Input: dimensioned drawing with shaded views. Units: mm. Origin: part minimum x, y, z. Round coordinates to 2 decimals unless told otherwise and drop trailing zeros. Loops run counter-clockwise (first coordinate to the right, second up) from the corner with the lowest first, then second, coordinate; pieces in that order, holes last. Notation, with made-up numbers: (42, 61.5) - (97, 61.5) arc R17 ccw to (97, 70.5) - close; hole circle Ø10 at (31.25, -0.75). An arc over 180 degrees is marked (long way). Answer as a JSON object with one key per item and string values. Group by question number.
Item 1: Line query: line 1 (Y direction, x = 29.5, z = 21.25) (1 decimal); line 2 (Y direction, x = 15.5, z = 11.75); line 3 (Y direction, x = 2.5, z = 3.5). Output: solid intervals per line, ascending.
Item 2: First-contact query: pin 1 (1.5 mm diameter, centred on x = 25.5, z = 8, fed in from +Y); pin 2 (4.5 mm diameter, centred on x = 27, z = 16, fed in from -Y); pin 3 (2 mm diameter, centred on x = 5, z = 12.5, fed in from +Y) (1 decimal). Flat tips, straight axial feed; report the tip coordinate or a pass-through.
Item 3: Section D-D (y = 5). Return the cut outline in (x, z), plus the area to 3 significant figures.
Item 4: Section C-C (x = 13). Return the cut outline in (y, z) (1 decimal), plus the area to 3 significant figures.
Item 5: Section B-B (z = 10.5). Return the cut outline in (x, y) (1 decimal), plus the area to 3 significant figures.
Item 6: Section A-A (x = 24). Return the cut outline in (y, z).
Item 7: Draft query along Y for the marked faces 1, 2 and 3. Return one class per face: released by +Y, released by -Y, zero draft, split by the parting line, or undercut.
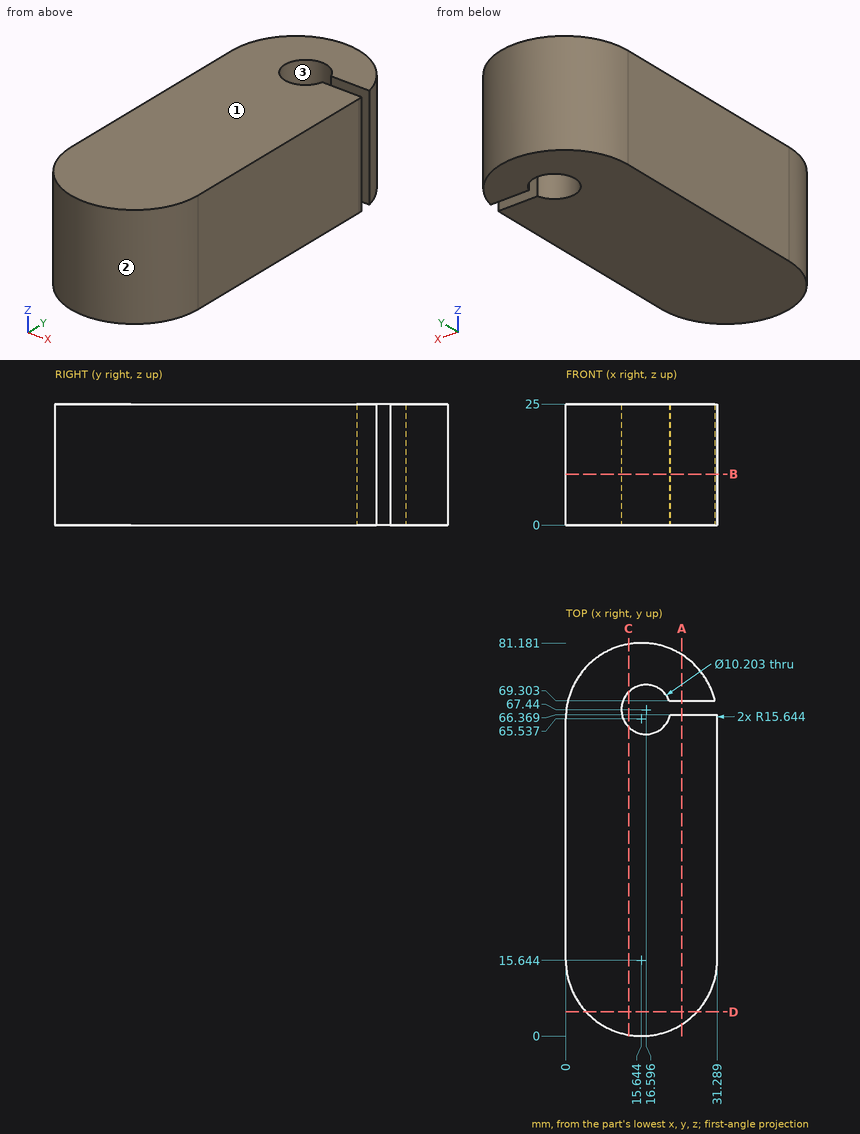
Values:
{
 "1": {"line 1": "y = 8.4 to 66.4, 69.3 to 72.8", "line 2": "y = 0 to 62.46, 72.42 to 81.18", "line 3": "y = 7.16 to 74.02"},
 "2": {"pin 1": "stops at y = 78.26", "pin 2": "stops at y = 2.92", "pin 3": "stops at y = 77.9"},
 "3": {"outline": "(4.18, 0) - (27.11, 0) - (27.11, 25) - (4.18, 25) - close", "area": "573 mm^2"},
 "4": {"outline": "(0.2, 0) - (63.8, 0) - (63.8, 25) - (0.2, 25) - close; (71.1, 0) - (81, 0) - (81, 25) - (71.1, 25) - close", "area": "1,840 mm^2"},
 "5": {"outline": "(0, 15.6) arc R15.6 ccw to (31.3, 15.6) - (31.3, 65.5) arc R15.6 ccw to (31.3, 66.4) - (21.6, 66.4) arc R5.1 cw (long way) to (21.3, 69.3) - (30.8, 69.3) arc R15.6 ccw to (0, 65.5) - close", "area": "2,220 mm^2"},
 "6": {"outline": "(2.42, 0) - (66.37, 0) - (66.37, 25) - (2.42, 25) - close; (69.3, 0) - (78.76, 0) - (78.76, 25) - (69.3, 25) - close"},
 "7": {"face 1": "zero draft", "face 2": "released by -Y", "face 3": "undercut"}
}
